Work out the finished part from the listing and answer in its coordinate system (mm). A direction names the side the tool comes from. Coordinates: 2 decimals unless noted, no trailing zeros. Write each loop counter-clockwise with the first axis right and the second up, starting at its lowest first coordinate (ties: lowest second). Pieces come first, ordered by that corner, then holes. Notation, with made-up numbers: (88, 54) - (136, 54) arc R28 ccw to (136, 78) - close; hole circle Ø7 at (-22.75, 54). An arc over 180 degrees is marked (long way). Use a Markdown table: item, result. Add a question column.
(1) For a pull along X with two mould halves and no side action, classify faces 3 (the face through (15.079, 7.605, -64.847)), 4 (the face through (-4.25, 7.4, -17.77)), 5 (the face through (224.771, 7, -70)) as released by +X, released by -X, zero draft, split by the parting line, or undercut.
(2) Find the intervals of material crossed by line 1 (X direction, y = 10.5, z = -65); line 2 (Z direction, x = 119, y = 2.75); line 3 (X direction, y = 14.5, z = -197), in increasing order. Write a range as from..to.
(3) A tool of negligible diameter and unlimited length cuts with its end or side. For faces 1 (the face through (19.812, 7.605, -151.817)), 2 (the face through (195, 7, -188.749)), from which of +Z, -Z, +X, -X, +Y, -Y can it reach the whole face along a straight path? Write none if from no direction.
(4) The part is cut by section C-C, the plane x = 118.5. Give the vertices of the cut face in (y, z), then the cut area to 3 significant figures.
(5) The part is cut by section D-D, the plane z = -117. Give the vertices of the cut face in (x, y), then the cut area to 3 significant figures.
(6) Given pin 1 Ø7.5 at (y, z) = (5.5, -219) entering from +X; pin 2 Ø4.5 at (x, y) = (199, 5.5) entering from -Z, each flat-ended and moving along its own axis, determine where each tip first touches the part or whether it passes through.
(7) The part is cut by section B-B, the plane y = 10.5. Give the vertices of the cut face in (x, z), then the cut area to 3 significant figures.
(8) The part is cut by section A-A, the plane x = 69. Give the vertices of the cut face in (y, z).
Solid Edge part; units mm, degrees
sketch "Sketch1" plane through (0, 0, 0) normal (0, -1, 0) x (1, 0, 0)
  line L0 (-75.229, -248.7494) -> (224.771, -248.7494)
  line L1 (224.771, -248.7494) -> (224.771, 51.2506)
  line L2 (224.771, 51.2506) -> (-75.229, 51.2506)
  line L3 (-75.229, 51.2506) -> (-75.229, -248.7494)
  dimension "D1" = 75.229
  dimension "D2" = 224.771
extrude "Protrusion1" add sketch "Sketch1" against normal blind 15
sketch "Sketch2" plane through (-15.229, 15, 1.2506) normal (0, 1, 0) x (-1, 0, 0)
  circle A0 centre (-34, -161) radius 8
  circle A1 centre (-34, -59) radius 8
  circle A2 centre (-136, -161) radius 8
  circle A3 centre (-85, -110) radius 20.5
  circle A4 centre (-136, -59) radius 8
extrude "Cutout1" cut sketch "Sketch2" against normal through all
sketch "Sketch3" plane through (49.771, 0, -73.7494) normal (0, -1, 0) x (-1, 0, 0)
  line L0 (-15, -125) -> (125, 15)
  line L1 (125, 15) -> (125, -125)
  line L2 (125, -125) -> (-15, -125)
  line L3 (-175, 115) -> (-115, 115)
  line L4 (-115, 115) -> (-115, 175)
  line L5 (-115, 175) -> (-175, 175)
  line L6 (-175, 175) -> (-175, 115)
  dimension "D1" = 175
  dimension "D2" = 175
  dimension "D3" = 125
extrude "Cutout2" cut sketch "Sketch3" against normal through all
properties material "Aluminum, 6061-T6"
Model answer:
| question | item | result |
|---|---|---|
| 1 | face 3 | undercut |
| 1 | face 4 | released by -X |
| 1 | face 5 | released by +X |
| 2 | line 1 | -51.48..15.39, 22.15..117.39, 124.15..224.77 |
| 2 | line 2 | -248.75..-167.55, -151.95..-65.55, -49.95..51.25 |
| 2 | line 3 | -75.23..164.77 |
| 3 | face 1 | +Y, -Y |
| 3 | face 2 | -Z, +X, +Y, -Y |
| 4 | outline | (0, -248.75) - (15, -248.75) - (15, -167.42) - (0, -167.42) - close; (0, -152.08) - (15, -152.08) - (15, -65.42) - (0, -65.42) - close; (0, -50.08) - (15, -50.08) - (15, 51.25) - (0, 51.25) - close |
| 4 | area | 4,040 mm^2 |
| 5 | outline | (-75.23, 0) - (51, 0) - (51, 15) - (-75.23, 15) - close; (88.54, 0) - (224.77, 0) - (224.77, 15) - (88.54, 15) - close |
| 5 | area | 3,940 mm^2 |
| 6 | pin 1 | x = 164.77 |
| 6 | pin 2 | z = -188.75 |
| 7 | outline | (-75.23, -248.75) - (164.77, -248.75) - (164.77, -188.75) - (224.77, -188.75) - (224.77, 51.25) - (64.77, 51.25) - (-75.23, -88.75) - close; hole circle Ø16 at (18.77, -159.75); hole circle Ø16 at (18.77, -57.75); hole circle Ø41 at (69.77, -108.75); hole circle Ø16 at (120.77, -159.75); hole circle Ø16 at (120.77, -57.75) |
| 7 | area | 74,500 mm^2 |
| 8 | outline | (0, -248.75) - (15, -248.75) - (15, -129.23) - (0, -129.23) - close; (0, -88.26) - (15, -88.26) - (15, 51.25) - (0, 51.25) - close |
